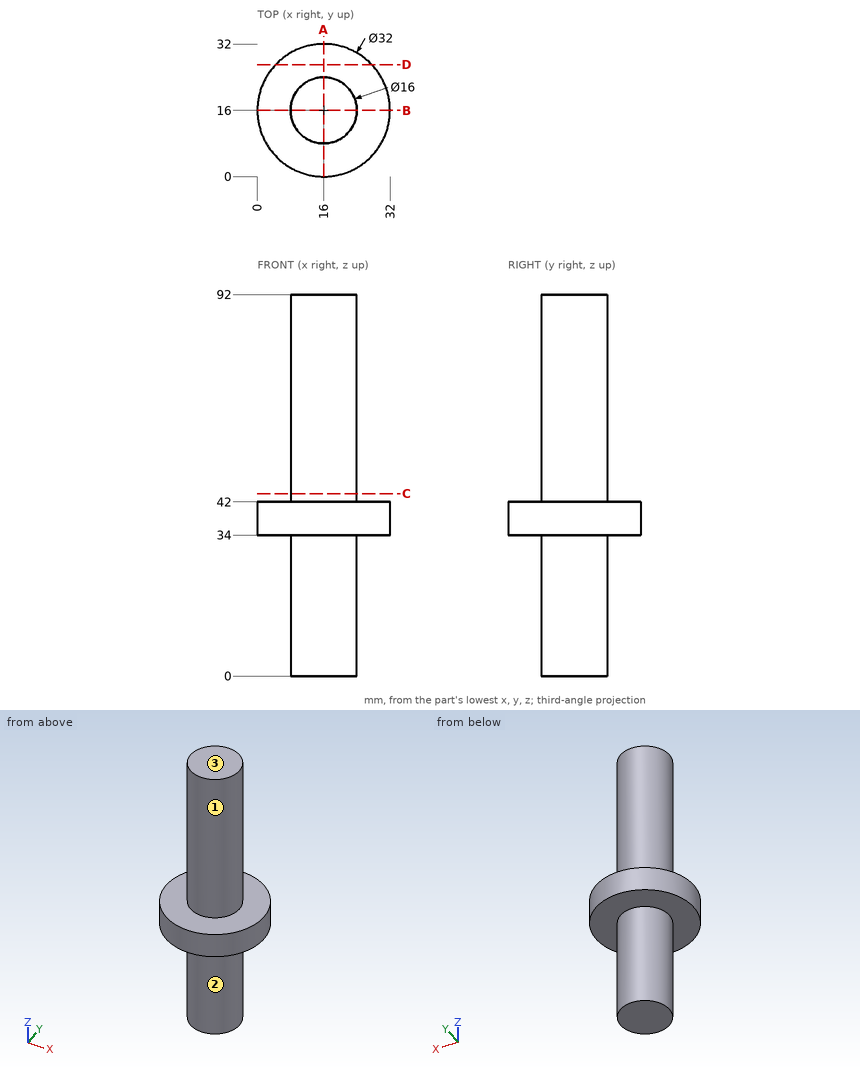
The drawing under review shows one solid part. Ordinate dimensions are in mm from its lowest x, y, z. A direction names the side the tool comes from. Coordinates: 2 decimals unless noted, no trailing zeros. Write each loop counter-clockwise with the first axis right and the second up, starting at its lowest first coordinate (ties: lowest second). Pieces come first, ordered by that corner, then holes. Notation, with made-up numbers: (85.25, -15.75) - (91.25, -15.75) arc R25 cw to (91.25, 22.25) - close; hole circle Ø8 at (-14, 0.5). An arc over 180 degrees is marked (long way). Answer in a Markdown table with one row per item. Add a question column.
Q1. We need section C-C, the plane z = 44. State the section outline as (x, y) points, and give its area (3 significant figures).
Q2. For P1, Ø2, axis at x = 12, y = 3.5, coming from the +Z side; P2, Ø5, axis at x = 4.5, z = 18.5, coming from the -Y side; P3, Ø10, axis at y = 21, z = 70.5, coming from the -X side; P4, Ø6, axis at y = 24, z = 70.5, coming from the +X side (3 decimals), all flat-tipped, find the tip position at first contact; note any pin that passes through.
Q3. We need section D-D, the plane y = 27. State the section outline as (x, z) points.
Q4. We need section A-A, the plane x = 16. State the section outline as (y, z) points.
Q5. Tool access review of the marked faces 1, 2 and 3: name each direction out of +Z, -Z, +X, -X, +Y, -Y from which nothing blocks a thin tool from reaching the whole face with its end or side.
Q6. For probe 1 along Z at (x, y) = (14, 24.5); probe 2 along Y at (x, z) = (15.5, 66.5); probe 3 along X at (y, z) = (16, 12), list the stretches that pass through material, from the lowest coordinate up.
Answer list:
| question | item | result |
|---|---|---|
| 1 | outline | circle Ø16 at (16, 16) |
| 1 | area | 201 mm2 |
| 2 | P1 | stops at z = 42 |
| 2 | P2 | passes through |
| 2 | P3 | stops at x = 8 |
| 2 | P4 | stops at x = 22.245 |
| 3 | outline | (4.38, 34) - (27.62, 34) - (27.62, 42) - (4.38, 42) - close |
| 4 | outline | (0, 34) - (8, 34) - (8, 0) - (24, 0) - (24, 34) - (32, 34) - (32, 42) - (24, 42) - (24, 92) - (8, 92) - (8, 42) - (0, 42) - close |
| 5 | face 1 | +Z |
| 5 | face 2 | -Z |
| 5 | face 3 | +Z, +X, -X, +Y, -Y |
| 6 | probe 1 | z = 34 to 42 |
| 6 | probe 2 | y = 8.02 to 23.98 |
| 6 | probe 3 | x = 8 to 24 |
